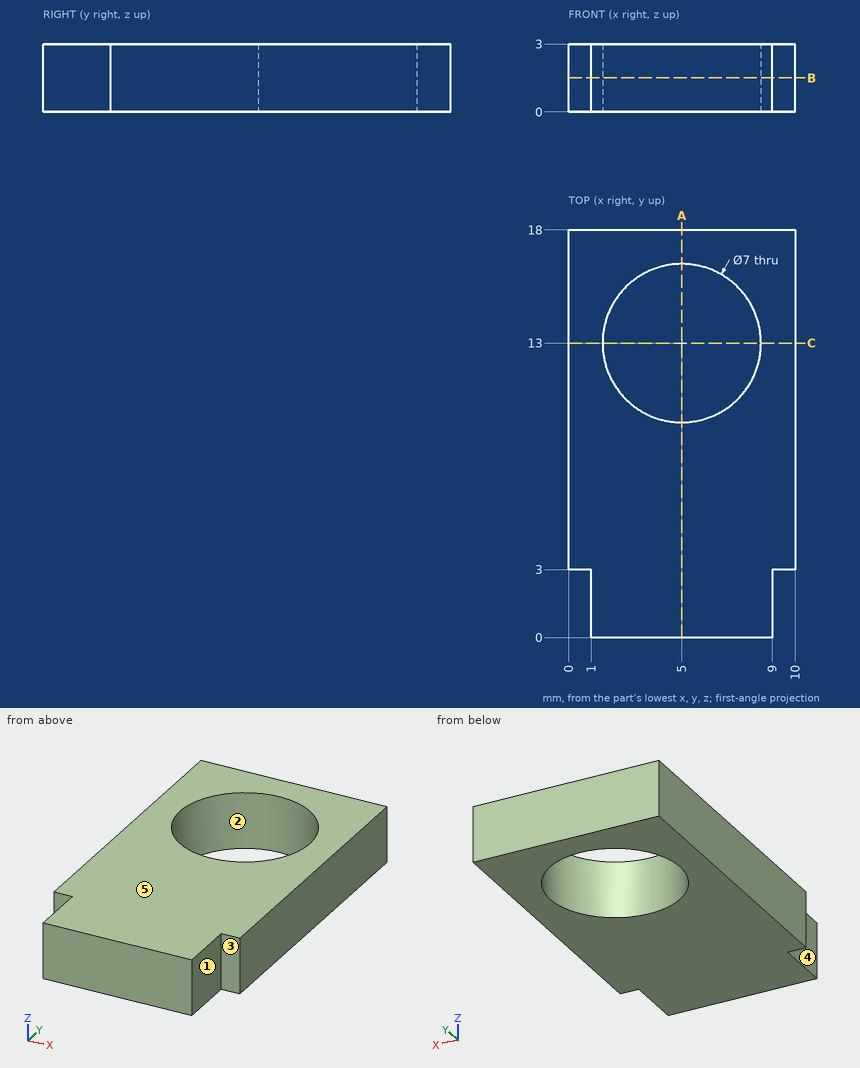
The drawing under review shows one solid part. Ordinate dimensions are in mm from its lowest x, y, z. A direction names the side the tool comes from. Round coordinates to 2 decimals unless told otherwise and drop trailing zeros. Loops run counter-clockwise (first coordinate to the right, second up) from the corner with the lowest first, then second, coordinate; pieces in that order, holes last. Notation, with made-up numbers: M 52,11.5 L 69,11.5 A11 cw 69,24.5 Z; hole C -20.75,47 d4. An arc over 180 degrees is marked long. Answer as CSV lines item,"result". Start each with the question number.
Item 1: Mouldability with a two-part tool opening along X and no side actions: class the marked faces 1, 2 and 3 as released by +X, released by -X, zero draft, split by the parting line, or undercut.
Item 2: Consider section A-A (x = 5). Write out the cut boundary in (y, z), then the cut area to 3 significant figures.
Item 3: Consider section B-B (z = 1.5). Write out the cut boundary in (x, y).
Item 4: Insertion check: P1, Ø1.5, axis at x = 3.5, y = 10, coming from the +Z side; P2, Ø0.8, axis at x = 9.5, z = 1, coming from the -Y side. Each pin has a flat end and moves straight along its axis. Give the tip position at first contact, or say it passes through.
Item 5: Wall thickness on line 1 (Y direction, x = 5, z = 1.85); line 2 (X direction, y = 11.25, z = 2.05); line 3 (X direction, y = 10.75, z = 1.7): over which ranges is each line inside the solid? List them lowest first. Write a range as [from, to].
Item 6: Consider section C-C (y = 13). Write out the cut boundary in (x, z), then the cut area to 3 significant figures.
Item 7: For the marked faces 4 and 5, list the 3-axis set-ups (+Z, -Z, +X, -X, +Y, -Y) from which the entire face can be reached by the end or side of a thin tool; tool diameter is ignored.
Answer:
1,face 1,"released by +X"
1,face 2,"undercut"
1,face 3,"zero draft"
2,outline,"M 0,0 L 9.5,0 L 9.5,3 L 0,3 Z; M 16.5,0 L 18,0 L 18,3 L 16.5,3 Z"
2,area,"33.0 mm^2"
3,outline,"M 0,3 L 1,3 L 1,0 L 9,0 L 9,3 L 10,3 L 10,18 L 0,18 Z; hole C 5,13 d7"
4,P1,"stops at z = 3"
4,P2,"stops at y = 3"
5,line 1,"y = [0, 9.5], [16.5, 18]"
5,line 2,"x = [0, 1.97], [8.03, 10]"
5,line 3,"x = [0, 2.32], [7.68, 10]"
6,outline,"M 0,0 L 1.5,0 L 1.5,3 L 0,3 Z; M 8.5,0 L 10,0 L 10,3 L 8.5,3 Z"
6,area,"9.00 mm^2"
7,face 4,"+Z, -Z, -X, -Y"
7,face 5,"+Z, +X, -X, +Y, -Y"
